```python
from build123d import *

# Parameters (mm, degrees)
SKETCH1_R           = 160
BOSS_EXTRUDE1_DEPTH = 6
CUT_EXTRUDE1_DEPTH  = 368.744476505
CUT_EXTRUDE2_DEPTH  = 368.744476505
SKETCH7_R           = 1.75
CUT_EXTRUDE3_DEPTH  = 368.744476505


with BuildPart() as part:
    # Sketch1 → Boss-Extrude1 (new body)
    with BuildSketch(Plane(origin=(0, 0, 0), x_dir=(1, 0, 0), z_dir=(0, 1, 0))):
        with Locations(Location((-100, 100, 0), (0, 0, 270))):
            Circle(SKETCH1_R)
    extrude(amount=BOSS_EXTRUDE1_DEPTH)

    # Sketch3 → Cut-Extrude1 (cut, through all)
    with BuildSketch(Plane.XZ):
        Polygon((-22.218254069, -227.279220614), (-46.966991411, -202.530483272), (2.530483272, -153.033008589), (27.279220614, -177.781745931), align=None)
        Polygon((2.530483272, -46.966991411), (27.279220614, -22.218254069), (-22.218254069, 27.279220614), (-46.966991411, 2.530483272), align=None)
        Polygon((-153.033008589, 2.530483272), (-177.781745931, 27.279220614), (-227.279220614, -22.218254069), (-202.530483272, -46.966991411), align=None)
        Polygon((-177.781745931, -227.279220614), (-153.033008589, -202.530483272), (-202.530483272, -153.033008589), (-227.279220614, -177.781745931), align=None)
    extrude(amount=-CUT_EXTRUDE1_DEPTH, mode=Mode.SUBTRACT)

    # Sketch4 → Cut-Extrude2 (cut, through all)
    with BuildSketch(Plane.XZ):
        Polygon((-31.23386553, -186.797357391), (-13.202642609, -168.76613447), (-74.013825791, -107.954951288), (-92.045048712, -125.986174209), align=None)
        Polygon((-125.986174209, -107.954951288), (-186.797357391, -168.76613447), (-168.76613447, -186.797357391), (-107.954951288, -125.986174209), align=None)
        Polygon((-107.954951288, -74.013825791), (-168.76613447, -13.202642609), (-186.797357391, -31.23386553), (-125.986174209, -92.045048712), align=None)
        Polygon((-74.013825791, -92.045048712), (-13.202642609, -31.23386553), (-31.23386553, -13.202642609), (-92.045048712, -74.013825791), align=None)
    extrude(amount=-CUT_EXTRUDE2_DEPTH, mode=Mode.SUBTRACT)

    # Sketch7 → Cut-Extrude3 (cut, through all)
    with BuildSketch(Plane.XZ):
        with Locations(Location((-149.002499936, -26.673026791, 0), (0, 0, 270))):
            Circle(SKETCH7_R)
        with Locations(Location((-148.578235868, -173.751237278, 0), (0, 0, 270))):
            Circle(SKETCH7_R)
        with Locations(Location((-140.163665171, -35.511861556, 0), (0, 0, 270))):
            Circle(SKETCH7_R)
        with Locations(Location((-164.912402513, -60.260598897, 0), (0, 0, 270))):
            Circle(SKETCH7_R)
        with Locations(Location((-173.751237278, -51.421764132, 0), (0, 0, 270))):
            Circle(SKETCH7_R)
        with Locations(Location((-173.326973209, -149.002499936, 0), (0, 0, 270))):
            Circle(SKETCH7_R)
        with Locations(Location((-164.488138444, -140.163665171, 0), (0, 0, 270))):
            Circle(SKETCH7_R)
        with Locations(Location((-139.739401103, -164.912402513, 0), (0, 0, 270))):
            Circle(SKETCH7_R)
        with Locations(Location((-26.673026791, -50.997500064, 0), (0, 0, 270))):
            Circle(SKETCH7_R)
        with Locations(Location((-35.511861556, -59.836334829, 0), (0, 0, 270))):
            Circle(SKETCH7_R)
        with Locations(Location((-60.260598897, -35.087597487, 0), (0, 0, 270))):
            Circle(SKETCH7_R)
        with Locations(Location((-51.421764132, -26.248762722, 0), (0, 0, 270))):
            Circle(SKETCH7_R)
        with Locations(Location((-50.997500064, -173.326973209, 0), (0, 0, 270))):
            Circle(SKETCH7_R)
        with Locations(Location((-59.836334829, -164.488138444, 0), (0, 0, 270))):
            Circle(SKETCH7_R)
        with Locations(Location((-35.087597487, -139.739401103, 0), (0, 0, 270))):
            Circle(SKETCH7_R)
        with Locations(Location((-26.248762722, -148.578235868, 0), (0, 0, 270))):
            Circle(SKETCH7_R)
    extrude(amount=-CUT_EXTRUDE3_DEPTH, mode=Mode.SUBTRACT)


solid = part.part
```
Geometry check sheet. Reference: the model listing, model coordinates, mm. Give positions to 0.01 mm unless a question says otherwise; leave off trailing zeros. Order: outer loops, then holes, each group sorted by start corner. A loop starts at its lowest first (then second) coordinate and runs counter-clockwise, first axis right, second up. Notation, with made-up numbers: (69.25, 4.5) - (119.25, 4.5) arc R36 cw to (119.25, 40.5) - close; hole circle Ø9 at (67, 78). An arc over 180 degrees is marked (long way). Write item = value, one per line. Start each with the question number.
1) Section check C-C (y = 2.75). Count the separate pieces of the cut face and the enclosed holes in it, then the cut area to 3 significant figures.
2) Gauge pin test, flat ends, axial feed: pin 1 Ø2 at (x, y) = (-88, 3) entering from -Z; pin 2 Ø3 at (y, z) = (2.5, -48) entering from -X; pin 3 Ø1 at (y, z) = (1.5, -163.5) entering from -X. Record the tip position at first contact, or that the pin passes through.
3) Scan lines: L1, parallel to X at y = 0.5, z = -123.5; L2, parallel to X at y = 1.5, z = -23; L3, parallel to Z at x = -209, y = 5. Record each from-to range of solid material in increasing order.
4) Section check B-B (x = -4.5). Enter the section's corners in (y, z).
5) Section check A-A (z = -207.5). Enter the section's corners in (x, y), then the cut area to 3 significant figures.
6) Draft check along Z on faces 1 (the flat face through (-98, 6, -102)), 2 (the flat face through (-43.18, 2.96, -138.79)). Enter one of: released by +Z, released by -Z, zero draft, split by the parting line, or undercut.
Geometry check:
q1.separate_pieces = 1
q1.enclosed_holes = 20
q1.area = 61,700 mm2
q2.pin_1 = -259.62
q2.pin_2 = -251.82
q2.pin_3 = -247.07
q3.L1 = -258.26 to -141.53, -110.44 to -89.56, -58.47 to 58.26
q3.L2 = -240.25 to -226.5, -158.97 to -41.03, 26.5 to 40.25
q3.L3 = -217.13 to -196.06, -159.5 to -40.5, -3.94 to 17.13
q4.outline = (0, -228.37) - (6, -228.37) - (6, -209.56) - (0, -209.56) - close; (0, -160.06) - (6, -160.06) - (6, -39.94) - (0, -39.94) - close; (0, 9.56) - (6, 9.56) - (6, 28.37) - (0, 28.37) - close
q5.outline = (-218.51, 0) - (-197.56, 0) - (-197.56, 6) - (-218.51, 6) - close; (-158, 0) - (-42, 0) - (-42, 6) - (-158, 6) - close; (-2.44, 0) - (18.51, 0) - (18.51, 6) - (-2.44, 6) - close
q5.area = 947 mm2
q6.face_1 = zero draft
q6.face_2 = undercut
